The listing builds one solid part. Answer for the finished solid, in the listing's coordinates (mm). A direction names the side the tool comes from. Give positions to 0.01 mm unless a question says otherwise; leave off trailing zeros. Loops run counter-clockwise (first coordinate to the right, second up) from the corner with the lowest first, then second, coordinate; pieces in that order, holes last.
Item 1: Section A-A, the plane y = 0.5 is taken. Give the vertices of the cut face in (x, z) (1 decimal).
Item 2: A tool of negligible diameter and unlimited length cuts with its end or side. For faces 4 (the face through (8, 0, -145)), 5 (the face through (8.31, 1.61, -87.58)), from which of +Z, -Z, +X, -X, +Y, -Y can it reach the whole face along a straight path? Write none if from no direction.
Item 3: The mould has two halves that part along Z. Classify faces 1 (the face through (21.41, 1.61, -189.05)), 2 (the face through (8, 3.175, -145)), 3 (the face through (-7.236, 1.61, -89.37)): pulls with the +Z half, pulls with the -Z half, needs draft (parallel to the pull), parting line crosses it, or undercut.
Item 4: Section B-B, the plane z = -247.5 is taken. Give the vertices of the cut face in (x, y) (3 decimals).
Item 5: Each of these flat-tipped pins is pushed along its axis until it touches: pin 1 Ø1.6 at (x, y) = (-26, 2) entering from +Z; pin 2 Ø1.5 at (y, z) = (2, -156.5) entering from -X. Where does it stop, or does it pass through?
Item 6: Consider line 1 along X through (y, z) = (2.6, -32); line 2 along X through (y, z) = (1.75, -89.5); line 3 along X through (y, z) = (0.45, -157.5). Determine where each line is inside the solid, lowest interval first.
Item 7: Section C-C, the plane x = 25.5 is taken. Give the vertices of the cut face in (y, z) (3 decimals), and give its area (3 significant figures).
from build123d import *

# Parameters (mm, degrees)
BOSS_EXTRUDE1_DEPTH = 3.175
CUT_EXTRUDE1_DEPTH  = 3.175
FILLET1_R           = 2.54
SKETCH3_W           = 44.45
SKETCH3_H           = 3.175
BOSS_EXTRUDE2_DEPTH = 4.7625
CUT_EXTRUDE2_DEPTH  = 375.826918736


with BuildPart() as part:
    # Sketch1 → Boss-Extrude1 (new body)
    with BuildSketch(Plane(origin=(0, 0, 0), x_dir=(1, 0, 0), z_dir=(0, 1, 0))):
        Polygon((0, 0), (-38.1, 0), (-5.08, 372.872), (0, 372.872), (8.89, 372.872), (38.1, 0), align=None)
    extrude(amount=BOSS_EXTRUDE1_DEPTH)

    # Sketch2 → Cut-Extrude1 (cut)
    with BuildSketch(Plane(origin=(0, 3.175, 0), x_dir=(1, 0, 0), z_dir=(0, 1, 0))):
        Polygon((13.379159589, 22.86), (0.937890665, 181.675502439), (-13.126152466, 22.86), align=None)
    extrude(amount=-CUT_EXTRUDE1_DEPTH, mode=Mode.SUBTRACT)

    # Fillet1
    fillet1_edges = [part.edges().sort_by_distance(p)[0] for p in [
        (-13.126152466, 1.5875, -22.86),
        (0.937890665, 1.5875, -181.675502439),
        (13.379159589, 1.5875, -22.86),
    ]]
    fillet(fillet1_edges, radius=FILLET1_R)

    # Sketch3 → Boss-Extrude2 (add)
    with BuildSketch(Plane.XY):
        with Locations((0, 1.5875)):
            Rectangle(SKETCH3_W, SKETCH3_H)
    extrude(amount=BOSS_EXTRUDE2_DEPTH)

    # Sketch4 → Cut-Extrude2 (cut, through all)
    with BuildSketch(Plane(origin=(0, 3.175, 0), x_dir=(1, 0, 0), z_dir=(0, 1, 0))):
        Polygon((-5.08, 372.872), (-34.29, 0), (-38.1, 0), align=None)
        Polygon((38.1, 0), (8.89, 372.872), (34.29, 0), align=None)
    extrude(amount=-CUT_EXTRUDE2_DEPTH, mode=Mode.SUBTRACT)


solid = part.part
Worked answers:
1. outline: (-34.3, 0) - (-5.1, -372.9) - (8.9, -372.9) - (34.3, 0) - (22.2, 0) - (22.2, 4.8) - (-22.2, 4.8) - (-22.2, 0) - close; hole (-12.9, -25.6) - (-1.7, -151.4) arc R2.5 ccw to (3.3, -151.3) - (13.2, -25.6) arc R2.5 ccw to (10.6, -22.9) - (-10.4, -22.9) arc R2.5 ccw to start
2. face 4: +Z, -Z, +X, -X, -Y
2. face 5: +Y, -Y
3. face 1: pulls with the -Z half
3. face 2: needs draft
3. face 3: undercut
4. outline: (-14.901, 0) - (17.43, 0) - (17.43, 3.175) - (-14.901, 3.175) - close
5. pin 1: stops at z = 0
5. pin 2: stops at x = -22.09
6. line 1: x = -31.78 to -12.32, 12.66 to 32.11
6. line 2: x = -27.28 to -7.22, 8.16 to 28.19
6. line 3: x = -21.95 to 23.56
7. outline: (0, -129.037) - (3.175, -129.037) - (3.175, 0) - (0, 0) - close
7. area: 410 mm2
